The model under review builds one solid part; all positions refer to its coordinate system, in mm. A direction names the side the tool comes from. Coordinates: 2 decimals unless noted, no trailing zeros. Write each loop counter-clockwise with the first axis right and the second up, starting at its lowest first coordinate (ties: lowest second). Pieces come first, ordered by that corner, then holes.
```python
from build123d import *

# Parameters (mm, degrees)
SALIENTE_EXTRUIR1_DEPTH = 15
CROQUIS2_W              = 5.35
CROQUIS2_H              = 27.5
CORTAR_EXTRUIR1_DEPTH   = 30
CROQUIS3_R              = 1.7
CORTAR_EXTRUIR2_DEPTH   = 30
REDONDEO1_R             = 10
REDONDEO2_R             = 2
CROQUIS4_R              = 2.95
CORTAR_EXTRUIR3_DEPTH   = 3
CORTAR_EXTRUIR4_DEPTH   = 3


with BuildPart() as part:
    # Croquis1 → Saliente-Extruir1 (new body)
    with BuildSketch(Plane.XY):
        with BuildLine():
            Line((9.25, -20.75), (-9.25, -20.75))
            Line((-9.25, -20.75), (-9.25, 20.75))
            ThreePointArc((-9.25, 20.75), (-3.831475452, 33.831475452), (9.25, 39.25))
            Line((9.25, 39.25), (9.25, 20.75))
            Line((9.25, 20.75), (9.25, -20.75))
        make_face()
    extrude(amount=SALIENTE_EXTRUIR1_DEPTH)

    # Croquis2 → Cortar-Extruir1 (cut)
    with BuildSketch(Plane(origin=(9.25, 0, 0), x_dir=(0, 0, -1), z_dir=(1, 0, 0))):
        with Locations((-7.5, -7)):
            Rectangle(CROQUIS2_W, CROQUIS2_H)
    extrude(amount=-CORTAR_EXTRUIR1_DEPTH, mode=Mode.SUBTRACT)

    # Croquis3 → Cortar-Extruir2 (cut)
    with BuildSketch(Plane.XY.offset(15)):
        with Locations((3.25, 1.75)):
            Circle(CROQUIS3_R)
        with Locations((-5.25, -16.75)):
            Circle(CROQUIS3_R)
    extrude(amount=-CORTAR_EXTRUIR2_DEPTH, mode=Mode.SUBTRACT)

    # Redondeo1
    redondeo1_edges = [part.edges().sort_by_distance(p)[0] for p in [
        (9.25, -20.75, 2.4125),
        (9.25, -20.75, 12.5875),
    ]]
    fillet(redondeo1_edges, radius=REDONDEO1_R)

    # Redondeo2
    redondeo2_edges = [part.edges().sort_by_distance(p)[0] for p in [
        (-3.831475452, 33.831475452, 15),
        (-9.25, 0, 0),
        (-3.831475452, 33.831475452, 0),
        (-9.25, 0, 15),
    ]]
    fillet(redondeo2_edges, radius=REDONDEO2_R)

    # Croquis4 → Cortar-Extruir3 (cut)
    with BuildSketch(Plane.XY.offset(15)):
        with Locations((3.25, 1.75)):
            Circle(CROQUIS4_R)
        with Locations((-5.25, -16.75)):
            Circle(CROQUIS4_R)
    extrude(amount=-CORTAR_EXTRUIR3_DEPTH, mode=Mode.SUBTRACT)

    # Croquis5 → Cortar-Extruir4 (cut)
    with BuildSketch(Plane(origin=(0, 0, 0), x_dir=(-1, 0, 0), z_dir=(0, 0, -1))):
        Polygon((-0.348814897, 3.425), (-3.25, 5.1), (-6.151185103, 3.425), (-6.151185103, 0.075), (-3.25, -1.6), (-0.348814897, 0.075), align=None)
        Polygon((5.25, -13.4), (2.348814897, -15.075), (2.348814897, -18.425), (5.25, -20.1), (8.151185103, -18.425), (8.151185103, -15.075), align=None)
    extrude(amount=-CORTAR_EXTRUIR4_DEPTH, mode=Mode.SUBTRACT)


solid = part.part
```
Item 1: Take a section at D-D, the plane z = 7.5. Write out the cut boundary in (x, y).
Solved:
outline: (-9.25, 6.75) - (9.25, 6.75) - (9.25, 39.25) arc R18.5 ccw to (-9.25, 20.75) - close
Item 2: For pin 1 (4 mm diameter, centred on x = -5.25, y = -16.75, fed in from -Z); pin 2 (2.5 mm diameter, centred on x = -4.5, z = 7, fed in from -Y); pin 3 (1.4 mm diameter, centred on y = -17.5, z = 2.5, fed in from +X), all flat-tipped, find the tip position at first contact; note any pin that passes through.
Solved:
pin 1: stops at z = 3
pin 2: stops at y = 6.75
pin 3: stops at x = 7.21
Item 3: Take a section at B-B, the plane y = 1.75. Write out the cut boundary in (x, z) (3 decimals), plus the area to 3 significant figures.
Solved:
outline: (-9.25, 2) arc R2 ccw to (-7.25, 0) - (0.349, 0) - (0.349, 3) - (1.55, 3) - (1.55, 4.825) - (-9.25, 4.825) - close; (-9.25, 10.175) - (1.55, 10.175) - (1.55, 12) - (0.3, 12) - (0.3, 15) - (-7.25, 15) arc R2 ccw to (-9.25, 13) - close; (4.95, 3) - (6.151, 3) - (6.151, 0) - (9.25, 0) - (9.25, 4.825) - (4.95, 4.825) - close; (4.95, 10.175) - (9.25, 10.175) - (9.25, 15) - (6.2, 15) - (6.2, 12) - (4.95, 12) - close
area: 129 mm2
Item 4: Machinability: for faces 1 (the face through (-2.436, -15.864, 13.521)), 2 (the face through (-3.9, -18.2, 3)), 3 (the face through (1, 9, 15)), which of the approach directions +Z, -Z, +X, -X, +Y, -Y give a long, thin tool a straight path to every point of the face, cutting with its end or side? Answer none if there is none.
Solved:
face 1: +Z
face 2: -Z
face 3: +Z, +X, -X, +Y, -Y
Item 5: Mouldability with a two-part tool opening along X and no side actions: class faces 4 (the face through (6.24, -17.9, 2.45)), 5 (the face through (-5, -19, 12)), 6 (the face through (0, 6.75, 8)) as pulls with the +X half, pulls with the -X half, needs draft (parallel to the pull), parting line crosses it, or undercut.
Solved:
face 4: pulls with the +X half
face 5: undercut
face 6: needs draft
Item 6: Take a section at A-A, the plane z = 3.75. Write out the cut boundary in (x, y).
Solved:
outline: (-9.25, -20.75) - (-0.75, -20.75) arc R10 ccw to (9.25, -10.75) - (9.25, 39.25) arc R18.5 ccw to (-9.25, 20.75) - close; hole circle Ø3.4 at (-5.25, -16.75); hole circle Ø3.4 at (3.25, 1.75)
Item 7: Take a section at C-C, the plane y = -16.75. Write out the cut boundary in (x, z) (3 decimals), plus the area to 3 significant figures.
Solved:
outline: (-9.25, 2) arc R2 ccw to (-8.151, 0.215) - (-8.151, 3) - (-6.95, 3) - (-6.95, 4.825) - (-9.25, 4.825) - close; (-9.25, 10.175) - (-6.95, 10.175) - (-6.95, 12) - (-8.2, 12) - (-8.2, 14.76) arc R2 ccw to (-9.25, 13) - close; (-3.55, 3) - (-2.349, 3) - (-2.349, 0) - (7.25, 0) - (7.25, 4.825) - (-3.55, 4.825) - close; (-3.55, 10.175) - (7.25, 10.175) - (7.25, 15) - (-2.3, 15) - (-2.3, 12) - (-3.55, 12) - close
area: 110 mm2
Item 8: To check wall thickness, follow line 1 along Z through (x, y) = (-0.75, -17) (3 decimals); line 2 along Z through (x, y) = (-6.5, -18) (3 decimals); line 3 along X through (y, z) = (-16.75, 13.75). State the ranges of each line that lie inside material, in increasing order.
Solved:
line 1: z = 0 to 4.825, 10.175 to 15
line 2: z = 3 to 4.825, 10.175 to 12
line 3: x = -9.1 to -8.2, -2.3 to 7.25
